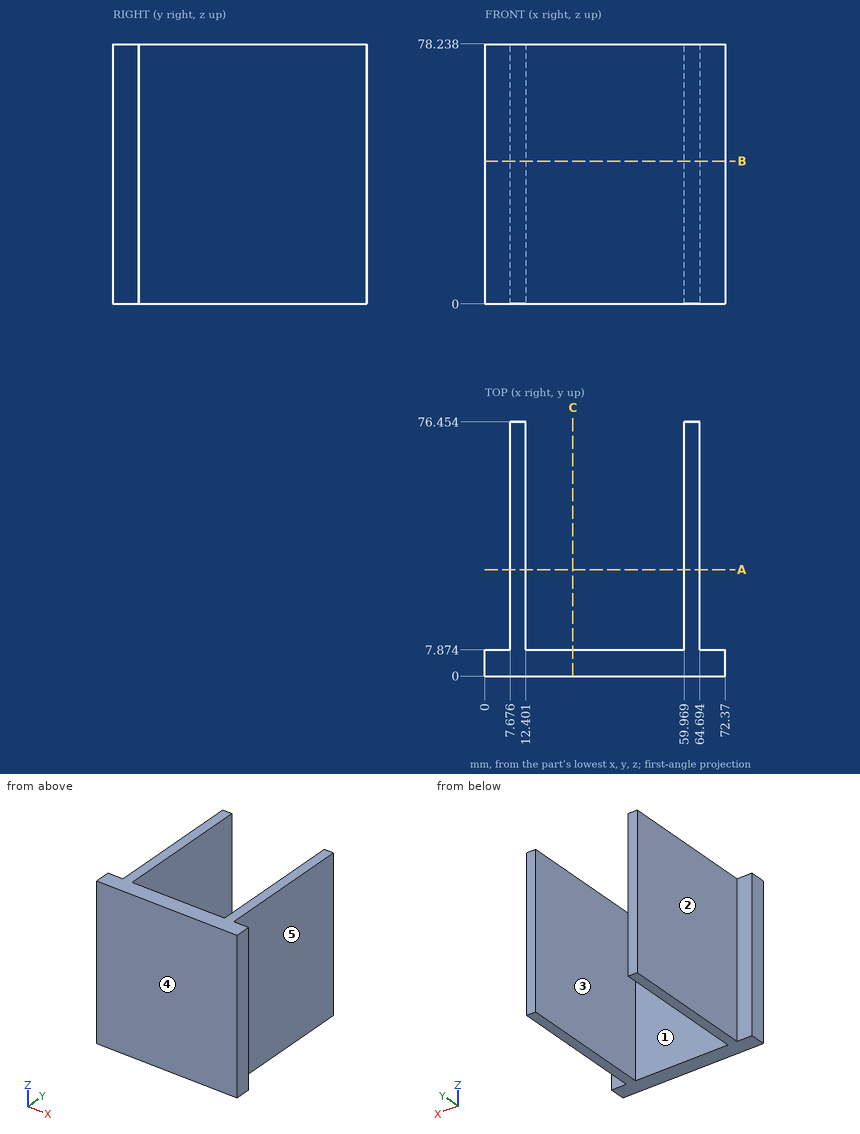
Can you work these out from the drawing? Everything is in mm from the part's minimum corner. A direction names the side the tool comes from. Give positions to 0.01 mm unless a question says otherwise; leave off trailing zeros. Order: outer loops, then holes, each group sorted by start corner. A loop starts at its lowest first (then second) coordinate and runs counter-clockwise, first axis right, second up. Notation, with made-up numbers: M 30,73.25 L 88,73.25 A20 cw 88,96.25 Z; hole C 3,43 d2. An arc over 180 degrees is marked long. Use a Markdown table: item, result. Add a question column.
Item 1: For the marked faces 1 and 2, which set-ups out of +Z, -Z, +X, -X, +Y, -Y let a thin tool reach every point of the face, with its end or its side?
Item 2: Suppose I cut it at A-A (y = 32). List the corners of the cut face in (x, z) for me (1 decimal).
Item 3: Will these pins go through, and if not, where does the flat tip stop? pin 1 (2 mm diameter, centred on x = 50, z = 55.5, fed in from +Y); pin 2 (1 mm diameter, centred on y = 36, z = 50.5, fed in from +X); pin 3 (2 mm diameter, centred on y = 60.5, z = 38, fed in from -X).
Item 4: If I drill on L1, parallel to X at y = 49, z = 57 (1 decimal); L2, parallel to Y at x = 39, z = 70, over which ranges is the centre line in solid material (lowest first)? Write a range as [from, to].
Item 5: We'd pull the mould along X, two halves only. Please class the marked faces 3, 4 and 5: +X half, -X half, draft (parallel to the pull), parting line (faces both ways), or undercut.
Item 6: Suppose I cut it at B-B (z = 43). List the corners of the cut face in (x, y) for me (1 decimal).
Item 7: Suppose I cut it at C-C (x = 26.5). List the corners of the cut face in (y, z) for me.
Answer sheet:
| question | item | result |
|---|---|---|
| 1 | face 1 | +Z, -Z, +Y |
| 1 | face 2 | +Z, -Z, -X, +Y |
| 2 | outline | M 7.7,0 L 12.4,0 L 12.4,78.2 L 7.7,78.2 Z; M 60,0 L 64.7,0 L 64.7,78.2 L 60,78.2 Z |
| 3 | pin 1 | stops at y = 7.87 |
| 3 | pin 2 | stops at x = 64.69 |
| 3 | pin 3 | stops at x = 7.68 |
| 4 | L1 | x = [7.7, 12.4], [60, 64.7] |
| 4 | L2 | y = [0, 7.87] |
| 5 | face 3 | undercut |
| 5 | face 4 | draft |
| 5 | face 5 | +X half |
| 6 | outline | M 0,0 L 72.4,0 L 72.4,7.9 L 64.7,7.9 L 64.7,76.5 L 60,76.5 L 60,7.9 L 12.4,7.9 L 12.4,76.5 L 7.7,76.5 L 7.7,7.9 L 0,7.9 Z |
| 7 | outline | M 0,0 L 7.87,0 L 7.87,78.24 L 0,78.24 Z |
